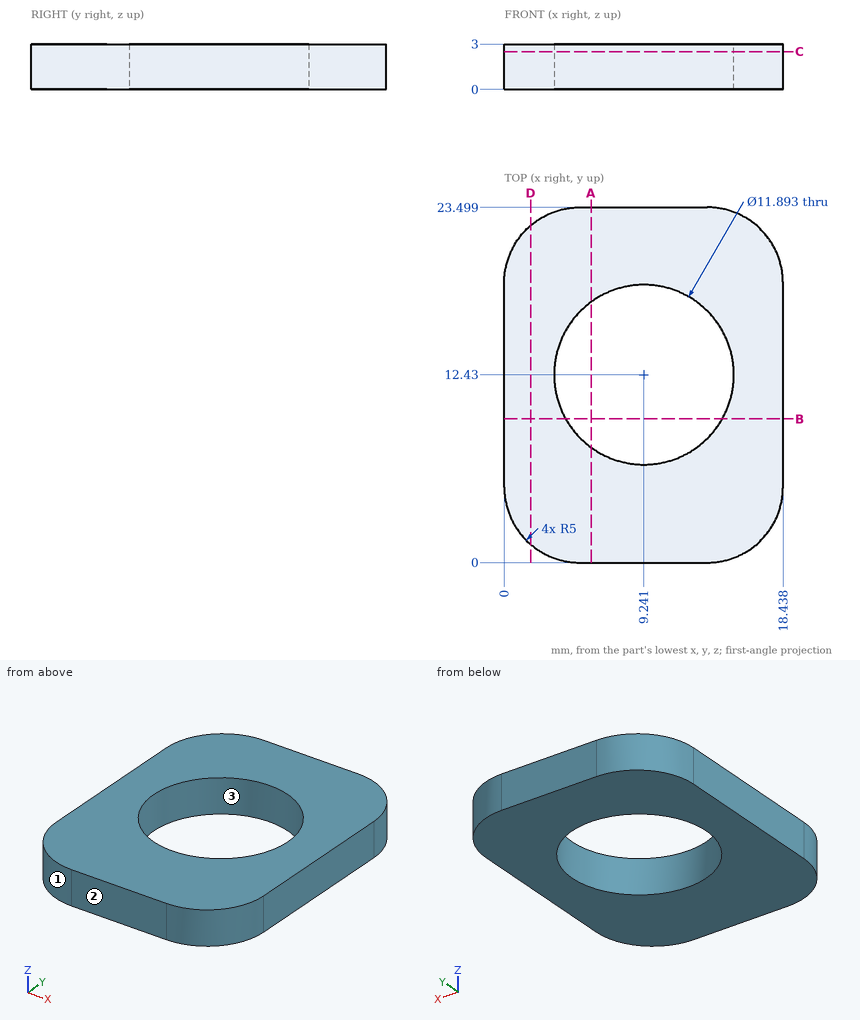
Here's the drawing with two shaded views (mm, measured from the low corner). I have some questions. Round coordinates to 2 decimals unless told otherwise and drop trailing zeros. Loops run counter-clockwise (first coordinate to the right, second up) from the corner with the lowest first, then second, coordinate; pieces in that order, holes last. Notation, with made-up numbers: (-9, 89.5) - (34, 89.5) arc R19 cw to (34, 114.5) - close; hole circle Ø11 at (-37.75, 26). An arc over 180 degrees is marked (long way). Use CSV: the item, a comma, the result in double quotes. Start each with the question number.
1) If we section it at A-A on x = 5.75: Write out the boundary of the cut face in (y, z) (1 decimal).
2) If we section it at D-D on x = 1.75: Write out the boundary of the cut face in (y, z).
3) If we section it at B-B on y = 9.5: Write out the boundary of the cut face in (x, z).
4) Please list where these lines run through material, in increasing order: probe 1 along X at (y, z) = (12.5, 1.1) (1 decimal); probe 2 along X at (y, z) = (15, 0.9) (1 decimal); probe 3 along Y at (x, z) = (13.25, 2.6) (1 decimal). Write a range as [from, to].
5) If we section it at C-C on z = 2.5: Write out the boundary of the cut face in (x, y), plus the area to 3 significant figures.
6) We'd pull the mould along X, two halves only. Please class the marked faces 1, 2 and 3: released by +X, released by -X, zero draft, split by the parting line, or undercut.
7) For pin 1 Ø5 at (x, y) = (15.5, 6.5) entering from -Z, with a flat end and sliding along its axis, tell me the tip position at first contact or that it passes through.
Geometry results:
1,outline,"(0, 0) - (7.6, 0) - (7.6, 3) - (0, 3) - close; (17.2, 0) - (23.5, 0) - (23.5, 3) - (17.2, 3) - close"
2,outline,"(1.2, 0) - (22.3, 0) - (22.3, 3) - (1.2, 3) - close"
3,outline,"(0, 0) - (4.07, 0) - (4.07, 3) - (0, 3) - close; (14.42, 0) - (18.44, 0) - (18.44, 3) - (14.42, 3) - close"
4,probe 1,"x = [0, 3.3], [15.2, 18.4]"
4,probe 2,"x = [0, 3.9], [14.6, 18.4]"
4,probe 3,"y = [0, 8], [16.8, 23.5]"
5,outline,"(0, 5) arc R5 ccw to (5, 0) - (13.44, 0) arc R5 ccw to (18.44, 5) - (18.44, 18.5) arc R5 ccw to (13.44, 23.5) - (5, 23.5) arc R5 ccw to (0, 18.5) - close; hole circle Ø11.89 at (9.24, 12.43)"
5,area,"301 mm2"
6,face 1,"released by -X"
6,face 2,"zero draft"
6,face 3,"undercut"
7,pin 1,"stops at z = 0"
